from build123d import *

# Parameters (mm, degrees)
SKETCH1_W               = 150
SKETCH1_H               = 200
BOSS_EXTRUDE1_DEPTH     = 5
SKETCH2_W               = 45
SKETCH2_H               = 50
CUT_EXTRUDE1_DEPTH      = 10
SKETCH3_W               = 35
SKETCH3_H               = 5
BOSS_EXTRUDE2_DEPTH     = 5
SKETCH5_W               = 5
SKETCH5_H               = 45
BOSS_EXTRUDE3_DEPTH     = 5
SKETCH6_W               = 45
SKETCH6_H               = 15
BOSS_EXTRUDE4_DEPTH     = 5
SKETCH7_W               = 5
SKETCH7_H               = 25
SKETCH7_H_2             = 50
BOSS_EXTRUDE5_DEPTH     = 5
SKETCH8_W               = 35
SKETCH8_H               = 250
CUT_EXTRUDE3_DEPTH      = 10
SKETCH9_R               = 2.1
CUT_EXTRUDE4_DEPTH      = 5
BOSS_EXTRUDE6_DEPTH     = 5
CUT_EXTRUDE5_DEPTH      = 5
SKETCH12_W              = 4.2
SKETCH12_H              = 5
CUT_EXTRUDE6_DEPTH      = 5
SKETCH13_W              = 5
SKETCH13_H              = 35
SKETCH13_H_2            = 45
BOSS_EXTRUDE7_DEPTH     = 5
SKETCH14_W              = 5
SKETCH14_H              = 25
CUT_EXTRUDE7_DEPTH      = 5
SKETCH15_W              = 20
SKETCH15_H              = 5
CUT_EXTRUDE8_DEPTH      = 5
SKETCH16_W              = 5
SKETCH16_H              = 25
CUT_EXTRUDE9_DEPTH      = 5
BOSS_EXTRUDE8_START     = -5
BOSS_EXTRUDE8_OUTLINE_R = 2.1
BOSS_EXTRUDE8_OUTLINE_W = 10
BOSS_EXTRUDE8_OUTLINE_H = 5
BOSS_EXTRUDE8_DEPTH     = 5
SKETCH18_W              = 10
SKETCH18_H              = 10
SKETCH18_W_2            = 5
SKETCH18_H_2            = 4
CUT_EXTRUDE10_DEPTH     = 5
CUT_EXTRUDE11_DEPTH     = 10
SKETCH20_W              = 10
SKETCH20_H              = 1.8
CUT_EXTRUDE13_DEPTH     = 10
SKETCH21_R              = 42.5
SKETCH21_R_2            = 3
CUT_EXTRUDE14_DEPTH     = 5
BOSS_EXTRUDE9_DEPTH     = 5
BOSS_EXTRUDE10_DEPTH    = 5
SKETCH24_R              = 2.1
BOSS_EXTRUDE11_DEPTH    = 5
SKETCH25_R              = 2.1
CUT_EXTRUDE15_DEPTH     = 5


# Read off the part's stored shape, not the designer's step: Boss-Extrude8
with BuildPart() as part:
    # Sketch1 → Boss-Extrude1 (new body)
    with BuildSketch(Plane.XY):
        with Locations((-75, 100)):
            Rectangle(SKETCH1_W, SKETCH1_H)
    extrude(amount=BOSS_EXTRUDE1_DEPTH)

    # Sketch2 → Cut-Extrude1 (cut)
    with BuildSketch(Plane.XY.offset(5)):
        with Locations((-22.5, 25)):
            Rectangle(SKETCH2_W, SKETCH2_H)
    extrude(amount=-CUT_EXTRUDE1_DEPTH, mode=Mode.SUBTRACT)

    # Sketch3 → Boss-Extrude2 (add)
    with BuildSketch(Plane(origin=(0, 0, 0), x_dir=(-1, 0, 0), z_dir=(0, 0, -1))):
        with Locations((65, 202.5)):
            Rectangle(SKETCH3_W, SKETCH3_H)
    extrude(amount=-BOSS_EXTRUDE2_DEPTH)

    # Sketch5 → Boss-Extrude3 (add)
    with BuildSketch(Plane.XY.offset(5)):
        Polygon((-50, 0), (-150, 0), (-150, -50), (-130, -50), (-130, -45), (-110, -45), (-110, -50), (-90, -50), (-90, -45), (-70, -45), (-70, -50), (-50, -50), (-50, -5), align=None)
        with Locations((-47.5, -27.5)):
            Rectangle(SKETCH5_W, SKETCH5_H)
    extrude(amount=-BOSS_EXTRUDE3_DEPTH)

    # Sketch6 → Boss-Extrude4 (add)
    with BuildSketch(Plane.XY.offset(5)):
        with Locations((-22.5, 42.5)):
            Rectangle(SKETCH6_W, SKETCH6_H)
    extrude(amount=-BOSS_EXTRUDE4_DEPTH)

    # Sketch7 → Boss-Extrude5 (add)
    with BuildSketch(Plane(origin=(0, 0, 0), x_dir=(-1, 0, 0), z_dir=(0, 0, -1))):
        with Locations((152.5, 27.5)):
            Rectangle(SKETCH7_W, SKETCH7_H)
        with Locations((152.5, 130)):
            Rectangle(SKETCH7_W, SKETCH7_H_2)
    extrude(amount=-BOSS_EXTRUDE5_DEPTH)

    # Sketch8 → Cut-Extrude3 (cut)
    with BuildSketch(Plane(origin=(0, 0, 0), x_dir=(-1, 0, 0), z_dir=(0, 0, -1))):
        with Locations((137.5, 75)):
            Rectangle(SKETCH8_W, SKETCH8_H)
    extrude(amount=-CUT_EXTRUDE3_DEPTH, mode=Mode.SUBTRACT)

    # Sketch9 → Cut-Extrude4 (cut)
    with BuildSketch(Plane.XY.offset(5)):
        with Locations((-72.5, 202.5)):
            Circle(SKETCH9_R)
    extrude(amount=-CUT_EXTRUDE4_DEPTH, mode=Mode.SUBTRACT)

    # Sketch10 → Boss-Extrude6 (add)
    with BuildSketch(Plane.XY.offset(5)):
        with BuildLine():
            Line((-76.830127019, 205), (-68.169872981, 205))
            ThreePointArc((-68.169872981, 205), (-72.5, 207.5), (-76.830127019, 205))
        make_face()
    extrude(amount=-BOSS_EXTRUDE6_DEPTH)

    # Sketch11 → Cut-Extrude5 (cut)
    with BuildSketch(Plane(origin=(0, 0, 0), x_dir=(-1, 0, 0), z_dir=(0, 0, -1))):
        with BuildLine():
            Line((21.830127019, 200), (13.169872981, 200))
            ThreePointArc((13.169872981, 200), (17.5, 197.5), (21.830127019, 200))
        make_face()
    extrude(amount=-CUT_EXTRUDE5_DEPTH, mode=Mode.SUBTRACT)

    # Sketch12 → Cut-Extrude6 (cut)
    with BuildSketch(Plane(origin=(0, 0, 0), x_dir=(-1, 0, 0), z_dir=(0, 0, -1))):
        Polygon((75, -40), (77.9, -40), (82.1, -40), (85, -40), (85, -30), (75, -30), align=None)
        with Locations((80, -42.5)):
            Rectangle(SKETCH12_W, SKETCH12_H)
    extrude(amount=-CUT_EXTRUDE6_DEPTH, mode=Mode.SUBTRACT)

    # Sketch13 → Boss-Extrude7 (add)
    with BuildSketch(Plane(origin=(-45, 0, 0), x_dir=(0, 0, -1), z_dir=(1, 0, 0))):
        with Locations((-2.5, 17.5)):
            Rectangle(SKETCH13_W, SKETCH13_H)
        with Locations((-2.5, -27.5)):
            Rectangle(SKETCH13_W, SKETCH13_H_2)
    extrude(amount=BOSS_EXTRUDE7_DEPTH)

    # Sketch14 → Cut-Extrude7 (cut)
    with BuildSketch(Plane(origin=(0, 0, 0), x_dir=(-1, 0, 0), z_dir=(0, 0, -1))):
        with Locations((42.5, -27.5)):
            Rectangle(SKETCH14_W, SKETCH14_H)
        with Locations((42.5, 17.5)):
            Rectangle(SKETCH14_W, SKETCH14_H)
    extrude(amount=-CUT_EXTRUDE7_DEPTH, mode=Mode.SUBTRACT)

    # Sketch15 → Cut-Extrude8 (cut)
    with BuildSketch(Plane(origin=(0, 0, 0), x_dir=(-1, 0, 0), z_dir=(0, 0, -1))):
        with Locations((20, 37.5)):
            Rectangle(SKETCH15_W, SKETCH15_H)
    extrude(amount=-CUT_EXTRUDE8_DEPTH, mode=Mode.SUBTRACT)

    # Sketch16 → Cut-Extrude9 (cut)
    with BuildSketch(Plane.XY.offset(5)):
        with Locations((-2.5, 102.5)):
            Rectangle(SKETCH16_W, SKETCH16_H)
        with Locations((-2.5, 162.5)):
            Rectangle(SKETCH16_W, SKETCH16_H)
    extrude(amount=-CUT_EXTRUDE9_DEPTH, mode=Mode.SUBTRACT)

    # Boss-Extrude8 outline → Boss-Extrude8 (add)
    with BuildSketch(Plane.XY.offset(5).offset(BOSS_EXTRUDE8_START)):
        with BuildLine():
            Line((0, 200), (0, 213.75))
            Line((0, 213.75), (-5, 213.75))
            Line((-5, 213.75), (-5, 222.5))
            Line((-5, 222.5), (-10, 222.5))
            Line((-10, 222.5), (-10, 227.5))
            Line((-10, 227.5), (-20, 227.5))
            Line((-20, 227.5), (-20, 222.5))
            Line((-20, 222.5), (-28.711001812, 222.5))
            ThreePointArc((-28.711001812, 222.5), (-66.079667431, 219.821548079), (-90, 248.65571123))
            Line((-90, 248.65571123), (-90, 282.5))
            Line((-90, 282.5), (-100.4, 282.5))
            Line((-100.4, 282.5), (-100.4, 277.5))
            Line((-100.4, 277.5), (-97.5, 277.5))
            Line((-97.5, 277.5), (-97.5, 269.3))
            Line((-97.5, 269.3), (-107.5, 269.3))
            Line((-107.5, 269.3), (-107.5, 277.5))
            Line((-107.5, 277.5), (-104.6, 277.5))
            Line((-104.6, 277.5), (-104.6, 282.5))
            Line((-104.6, 282.5), (-110, 282.5))
            Line((-110, 282.5), (-110, 287.5))
            Line((-110, 287.5), (-120, 287.5))
            Line((-120, 287.5), (-120, 200))
            Line((-120, 200), (-82.5, 200))
            Line((-82.5, 200), (-82.5, 205))
            Line((-82.5, 205), (-76.830127019, 205))
            ThreePointArc((-76.830127019, 205), (-72.5, 207.5), (-68.169872981, 205))
            Line((-68.169872981, 205), (-35, 205))
            Line((-35, 205), (-35, 200))
            Line((-35, 200), (-21.830127019, 200))
            ThreePointArc((-21.830127019, 200), (-17.5, 197.5), (-13.169872981, 200))
            Line((-13.169872981, 200), (0, 200))
        make_face()
        with Locations((-115, 225)):
            Circle(BOSS_EXTRUDE8_OUTLINE_R, mode=Mode.SUBTRACT)
        with Locations((-95, 225)):
            Rectangle(BOSS_EXTRUDE8_OUTLINE_W, BOSS_EXTRUDE8_OUTLINE_H, mode=Mode.SUBTRACT)
        with Locations((-17.5, 202.5)):
            Circle(BOSS_EXTRUDE8_OUTLINE_R, mode=Mode.SUBTRACT)
    extrude(amount=BOSS_EXTRUDE8_DEPTH)

    # Sketch18 → Cut-Extrude10 (cut)
    with BuildSketch(Plane.XY.offset(5)):
        with Locations((-15, 162.5)):
            Rectangle(SKETCH18_W, SKETCH18_H)
        with Locations((-7.5, 162.5)):
            Rectangle(SKETCH18_W_2, SKETCH18_H_2)
        with Locations((-7.5, 102.5)):
            Rectangle(SKETCH18_W_2, SKETCH18_H_2)
        Polygon((-10, 100.5), (-10, 104.5), (-10, 107.5), (-20, 107.5), (-20, 97.5), (-10, 97.5), align=None)
    extrude(amount=-CUT_EXTRUDE10_DEPTH, mode=Mode.SUBTRACT)

    # Sketch19 → Cut-Extrude11 (cut)
    with BuildSketch(Plane(origin=(0, 0, 0), x_dir=(-1, 0, 0), z_dir=(0, 0, -1))):
        Polygon((45, -25.4), (45, -29.6), (50, -29.6), (50, -32.5), (60, -32.5), (60, -22.5), (50, -22.5), (50, -25.4), align=None)
        Polygon((50, 12.5), (60, 12.5), (60, 22.5), (50, 22.5), (50, 19.6), (45, 19.6), (45, 15.4), (50, 15.4), align=None)
        Polygon((17.9, 40), (22.1, 40), (22.1, 45), (25, 45), (25, 55), (15, 55), (15, 45), (17.9, 45), align=None)
    extrude(amount=-CUT_EXTRUDE11_DEPTH, mode=Mode.SUBTRACT)

    # Sketch20 → Cut-Extrude13 (cut)
    with BuildSketch(Plane.XY.offset(5)):
        with Locations((-102.5, 268.4)):
            Rectangle(SKETCH20_W, SKETCH20_H)
    extrude(amount=-CUT_EXTRUDE13_DEPTH, mode=Mode.SUBTRACT)

    # Sketch21 → Cut-Extrude14 (cut)
    # profile 1 of 2: a face of its own
    with BuildSketch(Plane(origin=(0, 0, 0), x_dir=(-1, 0, 0), z_dir=(0, 0, -1))):
        with BuildLine():
            ThreePointArc((84.369317712, 282.5), (90.41624675, 270.644466464), (92.5, 257.5))
            Line((92.5, 257.5), (92.5, 282.5))
            Line((92.5, 282.5), (84.369317712, 282.5))
        make_face()
    # profile 2 of 2: a face of its own
    with BuildSketch(Plane(origin=(0, 0, 0), x_dir=(-1, 0, 0), z_dir=(0, 0, -1))):
        with Locations((50, 257.5)):
            Circle(SKETCH21_R)
        with Locations((50, 257.5)):
            Circle(SKETCH21_R_2, mode=Mode.SUBTRACT)
    extrude(amount=-CUT_EXTRUDE14_DEPTH, mode=Mode.SUBTRACT)

    # Sketch22 → Boss-Extrude9 (add)
    with BuildSketch(Plane(origin=(0, 0, 0), x_dir=(-1, 0, 0), z_dir=(0, 0, -1))):
        with BuildLine():
            Line((20, 222.5), (20, 227.396013553))
            ThreePointArc((20, 227.396013553), (22.834909521, 224.815020892), (25.890873098, 222.5))
            Line((25.890873098, 222.5), (20, 222.5))
        make_face()
    extrude(amount=-BOSS_EXTRUDE9_DEPTH)

    # Sketch23 → Boss-Extrude10 (add)
    with BuildSketch(Plane(origin=(0, 0, 0), x_dir=(-1, 0, 0), z_dir=(0, 0, -1))):
        with BuildLine():
            ThreePointArc((19.896013553, 227.5), (15.830207114, 232.227974871), (12.5, 237.5))
            Line((12.5, 237.5), (5, 237.5))
            Line((5, 237.5), (5, 227.5))
            Line((5, 227.5), (19.896013553, 227.5))
        make_face()
    extrude(amount=-BOSS_EXTRUDE10_DEPTH)

    # Sketch24 → Boss-Extrude11 (add)
    with BuildSketch(Plane(origin=(0, 0, 0), x_dir=(-1, 0, 0), z_dir=(0, 0, -1))):
        with Locations((115, 225)):
            Circle(SKETCH24_R)
    extrude(amount=-BOSS_EXTRUDE11_DEPTH)

    # Sketch25 → Cut-Extrude15 (cut)
    with BuildSketch(Plane(origin=(0, 0, 0), x_dir=(-1, 0, 0), z_dir=(0, 0, -1))):
        with Locations((108.5, 224.863108965)):
            Circle(SKETCH25_R)
    extrude(amount=-CUT_EXTRUDE15_DEPTH, mode=Mode.SUBTRACT)


solid = part.part
Read the model definition and answer for the solid it produces. Units are mm, in the model's axes. Round coordinates to 2 decimals unless told otherwise and drop trailing zeros. Write each loop counter-clockwise with the first axis right and the second up, starting at its lowest first coordinate (ties: lowest second). Pieces come first, ordered by that corner, then holes.
1. The part is cut by section A-A, the plane x = -53. Determine the outline of the cut face in (y, z), then the cut area to 3 significant figures.
2. Straight lines are drawn through the part: L1, parallel to X at y = 202.5, z = 3.7; L2, parallel to Y at x = -106, z = 1.9; L3, parallel to X at y = 223, z = 3.8. For each, find the intervals that lie inside material, in ascending order.
3. The part is cut by section B-B, the plane z = 2.8. State how many separate pieces and enclosed holes the cut face has, then the cut area to 3 significant figures.
4. Given pin 1 Ø2.5 at (x, z) = (-3, 3) entering from +Y; pin 2 Ø2.5 at (y, z) = (-47, 1.5) entering from -X; pin 3 Ø1.5 at (y, z) = (-3, 2.5) entering from +X, each flat-ended and moving along its own axis, determine where each tip first touches the part or whether it passes through.
Values:
1. outline: (-50, 0) - (-32.5, 0) - (-32.5, 5) - (-50, 5) - close; (-22.5, 0) - (12.5, 0) - (12.5, 5) - (-22.5, 5) - close; (22.5, 0) - (215.11, 0) - (215.11, 5) - (22.5, 5) - close
1. area: 1,230 mm2
2. L1: x = -120 to -74.6, -70.4 to -47.5, -35 to -19.6, -15.4 to 0
2. L2: y = -50 to 267.5, 277.5 to 282.5
2. L3: x = -120 to -109.47, -107.53 to -100, -90 to -74.82, -25.18 to -10
3. separate pieces: 1
3. enclosed holes: 5
3. area: 29,300 mm2
4. pin 1: stops at y = 213.75
4. pin 2: stops at x = -110
4. pin 3: stops at x = -50
